CAD build for the part. Positions are in the model's coordinates, mm. Face numbers are marked on the shaded views. A direction names the side the tool comes from. Give positions to 0.01 mm unless a question says otherwise; leave off trailing zeros. Write each loop counter-clockwise with the first axis right and the second up, starting at its lowest first coordinate (ties: lowest second). Pieces come first, ordered by that corner, then holes. Notation, with made-up numbers: M 36,61.25 L 57,61.25 A27 ccw 57,94.25 Z; hole C 22,-3.75 d6. An arc over 180 degrees is marked long. One line per question, with ' | ' between items. Start each with the question number.
1. Which spindle directions (+Z, -Z, +X, -X, +Y, -Y) get a long thin tool onto all of the face, cutting with end or side? Do the marked faces 1 and 2. Say none if no direction does.
2. Wall check: L1, parallel to X at y = 0, z = 0; L2, parallel to Z at x = -71, y = 0.85; L3, parallel to X at y = 1, z = -15.5. Give the ranges that are in metal, low to high.
3. Cut at D-D, the plane y = -18. Write the cut outline in (x, z), then the cut area to 3 significant figures.
4. Cut at C-C, the plane z = -11.5. Write the cut outline in (x, y), then the cut area to 3 significant figures.
5. Flat gauge pins, fed straight in: pin 1 (1 mm diameter, centred on x = 30, z = -2.5, fed in from +Y); pin 2 (10 mm diameter, centred on x = -27.5, z = -6, fed in from +Y); pin 3 (4.5 mm diameter, centred on x = 58, z = -1, fed in from -Y). Where does each tip first touch, or does it go through?
6. Cut at B-B, the plane x = 8.5. Write the cut outline in (y, z), then the cut area to 3 significant figures.
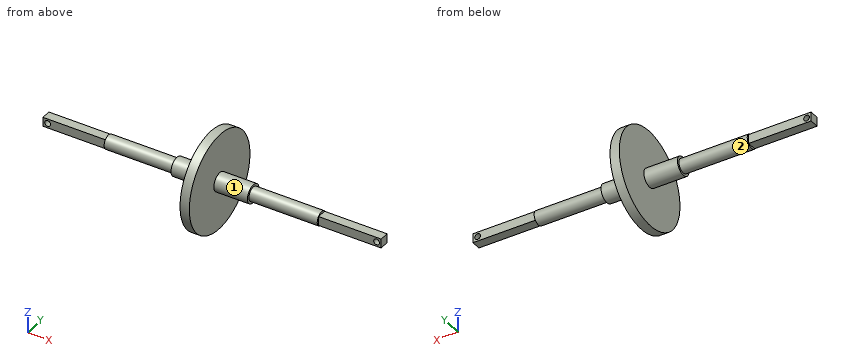
Solid Edge part; units mm, degrees
sketch "Sketch1" plane through (0, 0, 0) normal (1, 0, 0) x (0, 1, 0)
  circle A0 centre (0, 0) radius 21
extrude "Protrusion1" add sketch "Sketch1" along normal mid plane 4
sketch "Sketch2" plane through (-2, 0, 0) normal (-1, 0, 0) x (0, -1, 0)
  circle A0 centre (0, 0) radius 4
extrude "ProtrusiónExtruida_3" add sketch "Sketch2" along normal blind 14.5
sketch "Sketch3" plane through (-16.5, 0, 0) normal (-1, 0, 0) x (0, -1, 0)
  circle A0 centre (0, 0) radius 3
extrude "ProtrusiónExtruida_4" add sketch "Sketch3" along normal blind 29.5
sketch "Sketch4" plane through (-46, 0, 0) normal (-1, 0, 0) x (0, -1, 0)
  line L0 (2, -2) -> (2, 2)
  line L1 (2, 2) -> (-2, 2)
  line L2 (-2, 2) -> (-2, -2)
  line L3 (-2, -2) -> (2, -2)
extrude "ProtrusiónExtruida_5" add sketch "Sketch4" along normal blind 27
mirror "Mirror1" about plane through (0, 0, 0) normal (1, 0, 0) of "ProtrusiónExtruida_3", "ProtrusiónExtruida_4", "ProtrusiónExtruida_5"
sketch "Sketch5" plane through (-58, -2, 0) normal (0, -1, 0) x (-1, 0, 0)
  circle A0 centre (13, 0) radius 1.25
extrude "Cutout1" cut sketch "Sketch5" against normal up to next
mirror "Mirror2" about plane through (0, 0, 0) normal (1, 0, 0) of "Cutout1"
Here are the results:
1) face 1: +X | face 2: -X
2) L1: -73 to -72.25, -69.75 to 69.75, 72.25 to 73 | L2: -2 to -1.25, 1.25 to 2 | L3: -2 to 2
3) outline: M -2,-10.82 L 2,-10.82 L 2,10.82 L -2,10.82 Z | area: 86.5 mm^2
4) outline: M -2,-17.57 L 2,-17.57 L 2,17.57 L -2,17.57 Z | area: 141 mm^2
5) pin 1: y = 2.24 | pin 2: y = 2.83 | pin 3: y = -2
6) outline: C 0,0 d8 | area: 50.3 mm^2
